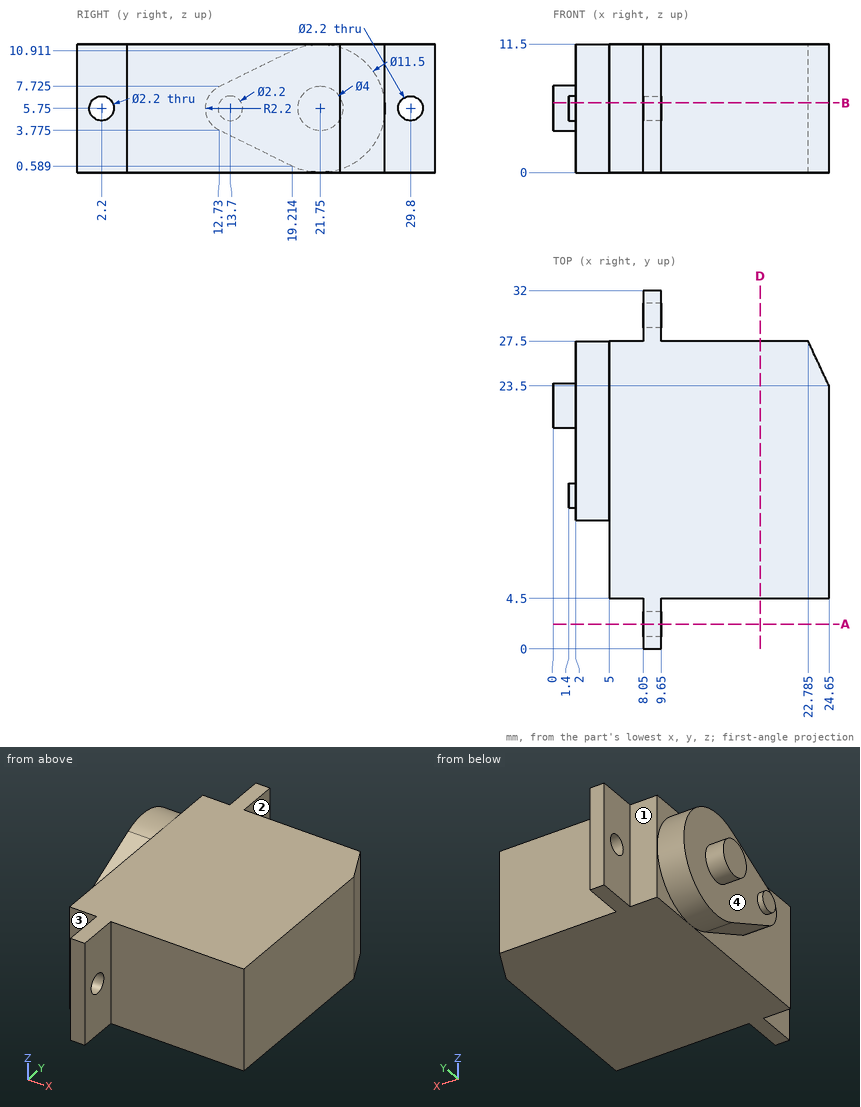
Geometry check sheet. Reference: drawing and pictorial views, mm from the part's lowest x, y, z. A direction names the side the tool comes from. Coordinates: 2 decimals unless noted, no trailing zeros. Order: outer loops, then holes, each group sorted by start corner. A loop starts at its lowest first (then second) coordinate and runs counter-clockwise, first axis right, second up. Notation, with made-up numbers: (-17.75, 51) - (-11.75, 51) arc R13 ccw to (-11.75, 71) - close; hole circle Ø10 at (62.5, -30). An arc over 180 degrees is marked (long way). Answer in a Markdown table with one row per item. Add a question column.
1) Material ranges on line 1 along Y through (x, z) = (8.6, 5.75); line 2 along X through (y, z) = (14.5, 9.5); line 3 along X through (y, z) = (18, 5.5), recorded low to high. Write a range as [from, to].
2) Cross-section at B-B, the plane z = 6.25. State how many separate pieces and enclosed holes the cut face has, then the cut area to 3 significant figures.
3) Cross-section at D-D, the plane x = 18.5. Record the cut outline in (y, z).
4) Cross-section at A-A, the plane y = 2.2. Record the cut outline in (x, z), then the cut area to 3 significant figures.
5) Set-up check for the marked faces 1, 2, 3 and 4: record each of +Z, -Z, +X, -X, +Y, -Y from which the full face is reachable in a straight line by a thin tool's end or side.
6) Gauge pin test, flat ends, axial feed: P1, Ø3.5, axis at x = 16.5, z = 3.5, coming from the -Y side; P2, Ø3.5, axis at y = 29, z = 6, coming from the -X side; P3, Ø1, axis at x = 12, z = 7, coming from the +Y side; P4, Ø5, axis at y = 2.5, z = 8, coming from the +X side. Record the tip position at first contact, or that the pin passes through.
Check result:
| question | item | result |
|---|---|---|
| 1 | line 1 | y = [0, 1.1], [3.3, 28.7], [30.9, 32] |
| 1 | line 2 | x = [5, 24.65] |
| 1 | line 3 | x = [2, 24.65] |
| 2 | separate pieces | 3 |
| 2 | enclosed holes | 0 |
| 2 | area | 513 mm² |
| 3 | outline | (4.5, 0) - (27.5, 0) - (27.5, 11.5) - (4.5, 11.5) - close |
| 4 | outline | (8.05, 0) - (9.65, 0) - (9.65, 4.65) - (8.05, 4.65) - close; (8.05, 6.85) - (9.65, 6.85) - (9.65, 11.5) - (8.05, 11.5) - close |
| 4 | area | 14.9 mm² |
| 5 | face 1 | +Z, -Z, -X, +Y |
| 5 | face 2 | +Z, -Z, +X, +Y |
| 5 | face 3 | +Z, -Z, -X, -Y |
| 5 | face 4 | -X |
| 6 | P1 | stops at y = 4.5 |
| 6 | P2 | stops at x = 2 |
| 6 | P3 | stops at y = 27.5 |
| 6 | P4 | stops at x = 24.65 |
